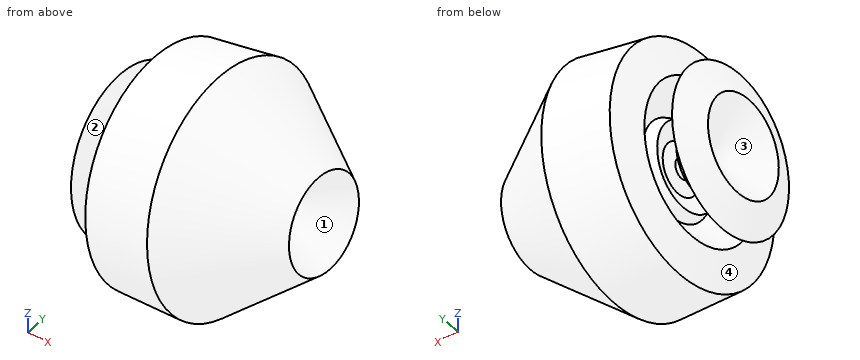
from build123d import *


with BuildPart() as f1:
    # F0 (on Front) → F1 (revolve)
    with BuildSketch(Plane.XZ):
        Polygon((-67.0393481851, -4.226393532), (-42.2639362514, -34.2483595014), (38.1832793355, -25.212623179), (-13.1163932383, 31.6250808537), (-35.8514748514, 42.9926253855), (-38.7662313879, 17.9257374257), (-19.9521857218, 0), (-27.3986887187, -4.226393532), (-21.2777052075, -15.0109836832), (-21.2777052075, -25.212623179), (-31.7708216608, -25.212623179), (-35.8514748514, -10.9303286299), (-48.0934418738, -4.226393532), (-60.3354126215, 17.9257374257), align=None)
        Polygon((-13.1163932383, 31.6250808537), (38.1832793355, -25.212623179), (78.9898335934, 11.8047548458), (9.6186883748, 51.153935492), (-35.8514748514, 42.9926253855), align=None)
    revolve(axis=Axis((-2.040328458, 0, -29.7304913402), (0.9937513025, 0, 0.1116169736)))


solid = f1.part
Build history of the part. All positions in model axes, mm. Face numbers are marked on the shaded views. A direction names the side the tool comes from. Round coordinates to 2 decimals unless told otherwise and drop trailing zeros. Use CSV: the item, a comma, the result in double quotes. Start each with the question number.
Q1. Which spindle directions (+Z, -Z, +X, -X, +Y, -Y) get a long thin tool onto all of the face, cutting with end or side? Do the marked faces 1 and 2. Say none if no direction does.
Q2. Mould opens along Z. For the marked faces 3 and 4 say: +Z half, -Z half, draft (parallel to the pull), parting line (faces both ways), or undercut.
Q3. Flat gauge pins, fed straight in: pin 1 Ø12 at (x, z) = (7.5, -48) entering from -Y; pin 2 Ø1.5 at (x, y) = (-18, -23.5) entering from -Z; pin 3 Ø3 at (x, y) = (24, 5.5) entering from +Z. Where does each tip first touch, or does it go through?
Q4. Drill centre lines: L1, parallel to Y at x = -19.5, z = -5; L2, parallel to Y at x = -24, z = -27; L3, parallel to Z at x = 75.5, y = 2.5. Where is each one in solid material? Low to high.
Solutions:
1,face 1,"+X"
1,face 2,"none"
2,face 3,"undercut"
2,face 4,"parting line"
3,pin 1,"stops at y = -77.16"
3,pin 2,"stops at z = -104.63"
3,pin 3,"stops at z = 43.65"
4,L1,"y = -72.03 to -17.31, -16.99 to 16.99, 17.31 to 72.03"
4,L2,"y = -76.13 to -39.6, -28.06 to -25.71, -4.67 to 4.67, 25.71 to 28.06, 39.6 to 76.13"
4,L3,"z = -61.92 to -46.12, 8.52 to 13.7"
